Autodesk Inventor part; units mm, degrees
ref_plane "YZ Plane" through (0, 0, 0) normal (1, 0, 0) x (0, 1, 0)
ref_plane "XZ Plane" through (0, 0, 0) normal (0, 1, 0) x (-1, 0, 0)
ref_plane "XY Plane" through (0, 0, 0) normal (0, 0, 1) x (1, 0, 0)
sketch "Sketch1" plane through (0, 0, 0) normal (0, 0, 1) x (1, 0, 0)
  circle A0 centre (0, 0) radius 50
  dimension "d0" = 100
extrude "Extrusion1" add sketch "Sketch1" along normal mid plane 75
sketch "Sketch2" plane through (0, 0, 37.5) normal (0, 0, 1) x (1, 0, 0)
  circle A0 centre (0, 0) radius 37.5
  dimension "d3" = 75
extrude "Extrusion2" cut sketch "Sketch2" against normal through all
sketch "Sketch4" plane through (0, 0, 0) normal (0, 0, 1) x (1, 0, 0)
  line L0 (25, -43.3013) -> (25, -52)
  line L1 (25, -52) -> (-25, -52)
  line L2 (-25, -52) -> (-25, -43.3013)
  arc A0 (-25, -43.3013) -> (25, -43.3013) centre (0, 0) ccw
  circle A1 centre (0, 0) radius 50
  line L3 (0, 0) -> (0, -66.2618) construction
  dimension "d22" = 50
  dimension "d24" = 90
  dimension "d25" = 50
  dimension "d26" = 52
extrude "Extrusion3" add sketch "Sketch4" along normal mid plane 50 contours L0 L1 L2 A0
sketch "Sketch6" plane through (-25, -52, 25) normal (0, -1, 0) x (1, 0, 0)
  circle A0 centre (25, -25) radius 20
  dimension "d27" = 40
extrude "Extrusion5" add sketch "Sketch6" along normal blind 10
properties material "ABS Plastic"
Build history of the part. All positions in model axes, mm. A direction names the side the tool comes from. Round coordinates to 2 decimals unless told otherwise and drop trailing zeros. Write each loop counter-clockwise with the first axis right and the second up, starting at its lowest first coordinate (ties: lowest second). Pieces come first, ordered by that corner, then holes. Notation, with made-up numbers: (-8, 82.5) - (21, 82.5) arc R24 cw to (21, 116.5) - close; hole circle Ø1 at (1, 58.5). An arc over 180 degrees is marked (long way). Write each question's results on one line, items separated by ' | '. Start each with the question number.
Item 1: Which spindle directions (+Z, -Z, +X, -X, +Y, -Y) get a long thin tool onto all of the face, cutting with end or side? Do faces 1 (the face through (-0.4, -50.5, -25)), 2 (the face through (25, -48, 0)), 3 (the face through (-25, -48, 0)), 4 (the face through (17, -52, -11)), 5 (the face through (-0.4, -50.5, 25)). Say none if no direction does.
Item 2: Mould opens along Y. For faces 6 (the face through (-4.336, -56.93, 19.524)), 7 (the face through (-4.88, 37.18, 0.52)), 8 (the face through (23.07, 44.36, -0.52)) say: pulls with the +Y half, pulls with the -Y half, needs draft (parallel to the pull), parting line crosses it, or undercut.
Item 3: Saw through at B-B (y = -30). Write the cut outline in (x, z).
Item 4: Saw through at C-C (z = 0). Write the cut outline in (x, y), and give its area (3 significant figures).
Item 5: Drop flat-ended pins along their axis: P1, Ø2.5, axis at y = -47, z = 2.5, coming from the +X side; P2, Ø1, axis at x = 28, z = 22, coming from the +Y side; P3, Ø10, axis at x = 2, z = -3.5, coming from the +Y side. Give the stop position or say it passes through.
Item 6: Saw through at A-A (x = 0). Write the cut outline in (y, z).
Item 7: Wall check: L1, parallel to Y at x = 0, z = -22; L2, parallel to Y at x = 0, z = -17.5; L3, parallel to X at y = 34, z = 29. Give the ranges that are in metal, low to high. Write a range as [from, to].
Item 8: Saw through at D-D (y = -2.5). Write the cut outline in (x, z), and give its area (3 significant figures).
Results are:
1) face 1: -Z, -Y | face 2: +Z, -Z, +X, -Y | face 3: +Z, -Z, -X, -Y | face 4: -Y | face 5: +Z, -Y
2) face 6: needs draft | face 7: undercut | face 8: parting line crosses it
3) outline: (-40, -37.5) - (-22.5, -37.5) - (-22.5, 37.5) - (-40, 37.5) - close; (22.5, -37.5) - (40, -37.5) - (40, 37.5) - (22.5, 37.5) - close
4) outline: (-25, -52) - (-20, -52) - (-20, -62) - (20, -62) - (20, -52) - (25, -52) - (25, -43.3) arc R50 ccw (long way) to (-25, -43.3) - close; hole circle Ø75 at (0, 0) | area: 4,040 mm²
5) P1: stops at x = 25 | P2: stops at y = 41.76 | P3: stops at y = 50
6) outline: (-62, -20) - (-52, -20) - (-52, -25) - (-50, -25) - (-50, -37.5) - (-37.5, -37.5) - (-37.5, 37.5) - (-50, 37.5) - (-50, 25) - (-52, 25) - (-52, 20) - (-62, 20) - close; (37.5, -37.5) - (50, -37.5) - (50, 37.5) - (37.5, 37.5) - close
7) L1: y = [-52, -37.5], [37.5, 50] | L2: y = [-62, -37.5], [37.5, 50] | L3: x = [-36.66, -15.82], [15.82, 36.66]
8) outline: (-49.94, -37.5) - (-37.42, -37.5) - (-37.42, 37.5) - (-49.94, 37.5) - close; (37.42, -37.5) - (49.94, -37.5) - (49.94, 37.5) - (37.42, 37.5) - close | area: 1,880 mm²
